Geometry check sheet. Reference: drawing and pictorial views, mm from the part's lowest x, y, z. A direction names the side the tool comes from. Coordinates: 2 decimals unless noted, no trailing zeros. Write each loop counter-clockwise with the first axis right and the second up, starting at its lowest first coordinate (ties: lowest second). Pieces come first, ordered by that corner, then holes. Notation, with made-up numbers: (69, -26.75) - (95, -26.75) arc R29 cw to (95, 8.25) - close; hole circle Ø9 at (79, 4.25). An arc over 180 degrees is marked (long way). Answer as CSV lines item,"result". Start each with the question number.
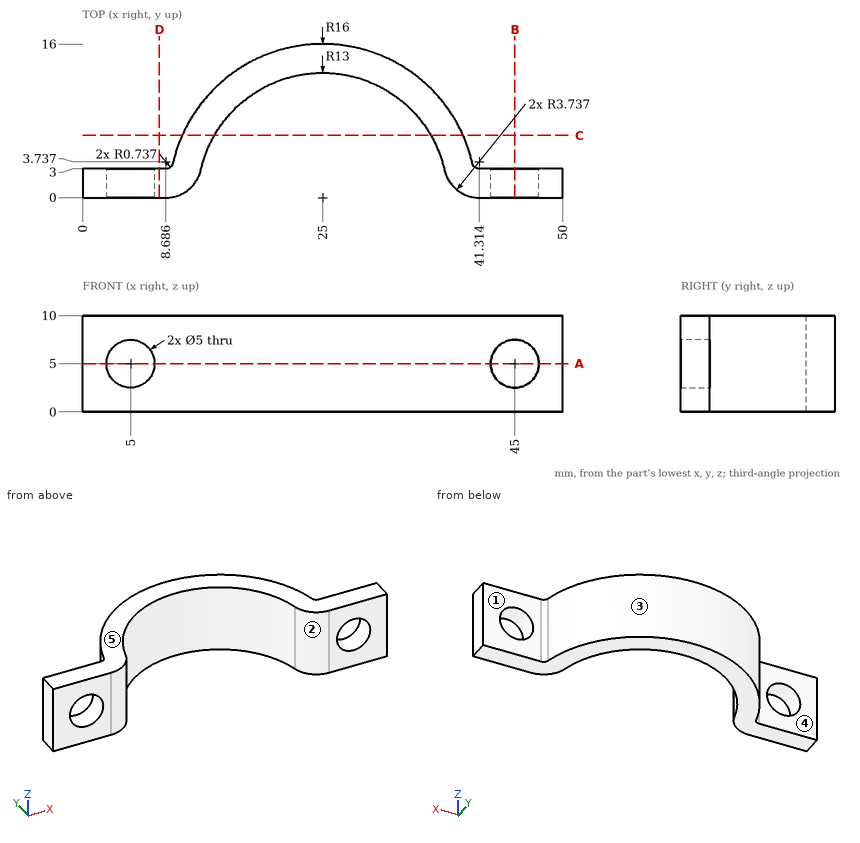
1. Cross-section at A-A (z = 5). Record the cut outline in (x, y), and give its area (3 significant figures).
2. Draft check along X on the marked faces 1, 2 and 3. Enter one of: pulls with the +X half, pulls with the -X half, needs draft (parallel to the pull), parting line crosses it, or undercut.
3. Cross-section at B-B (x = 45). Record the cut outline in (y, z), and give its area (3 significant figures).
4. Cross-section at D-D (x = 8). Record the cut outline in (y, z).
5. Access from +Z, -Z, +X, -X, +Y, -Y to the whole of each face (thin tool, end or side, straight path). Record for the marked faces 4 and 5.
6. Scan lines: line 1 along Z through (x, y) = (45, 1.9); line 2 along X through (y, z) = (1.1, 5) (1 decimal); line 3 along X through (y, z) = (0.9, 5). Record each from-to range of solid material in increasing order. Write a range as from..to.
7. Cross-section at C-C (y = 6.5). Record the cut outline in (x, z).
8. Depth check by flat-ended pin: P1, Ø5, axis at y = 7.5, z = 7.5, coming from the +X side; P2, Ø5, axis at x = 31.5, z = 8.5, coming from the +Y side; P3, Ø2, axis at y = 6.5, z = 6, coming from the -X side (1 decimal). Enter the tip coordinate at first touch or a pass-through.
Completed:
1,outline,"(0, 0) - (2.5, 0) - (2.5, 3) - (0, 3) - close; (7.5, 0) - (8.69, 0) arc R3.74 ccw to (12.33, 2.9) arc R13 cw to (37.67, 2.9) arc R3.74 ccw to (41.31, 0) - (42.5, 0) - (42.5, 3) - (41.31, 3) arc R0.74 cw to (40.6, 3.57) arc R16 ccw to (9.4, 3.57) arc R0.74 cw to (8.69, 3) - (7.5, 3) - close; (47.5, 0) - (50, 0) - (50, 3) - (47.5, 3) - close"
1,area,"157 mm2"
2,face 1,"needs draft"
2,face 2,"undercut"
2,face 3,"parting line crosses it"
3,outline,"(0, 0) - (3, 0) - (3, 2.5) - (0, 2.5) - close; (0, 7.5) - (3, 7.5) - (3, 10) - (0, 10) - close"
3,area,"15.0 mm2"
4,outline,"(0, 0) - (3, 0) - (3, 10) - (0, 10) - close"
5,face 4,"+Z, -Z, -X, +Y"
5,face 5,"+Z, +X, -X, +Y, -Y"
6,line 1,"z = 0..2.5, 7.5..10"
6,line 2,"x = 0..2.5, 7.5..11.3, 38.7..42.5, 47.5..50"
6,line 3,"x = 0..2.5, 7.5..11.12, 38.88..42.5, 47.5..50"
7,outline,"(10.38, 0) - (13.74, 0) - (13.74, 10) - (10.38, 10) - close; (36.26, 0) - (39.62, 0) - (39.62, 10) - (36.26, 10) - close"
8,P1,"stops at x = 40.2"
8,P2,"stops at y = 15.49"
8,P3,"stops at x = 10"
